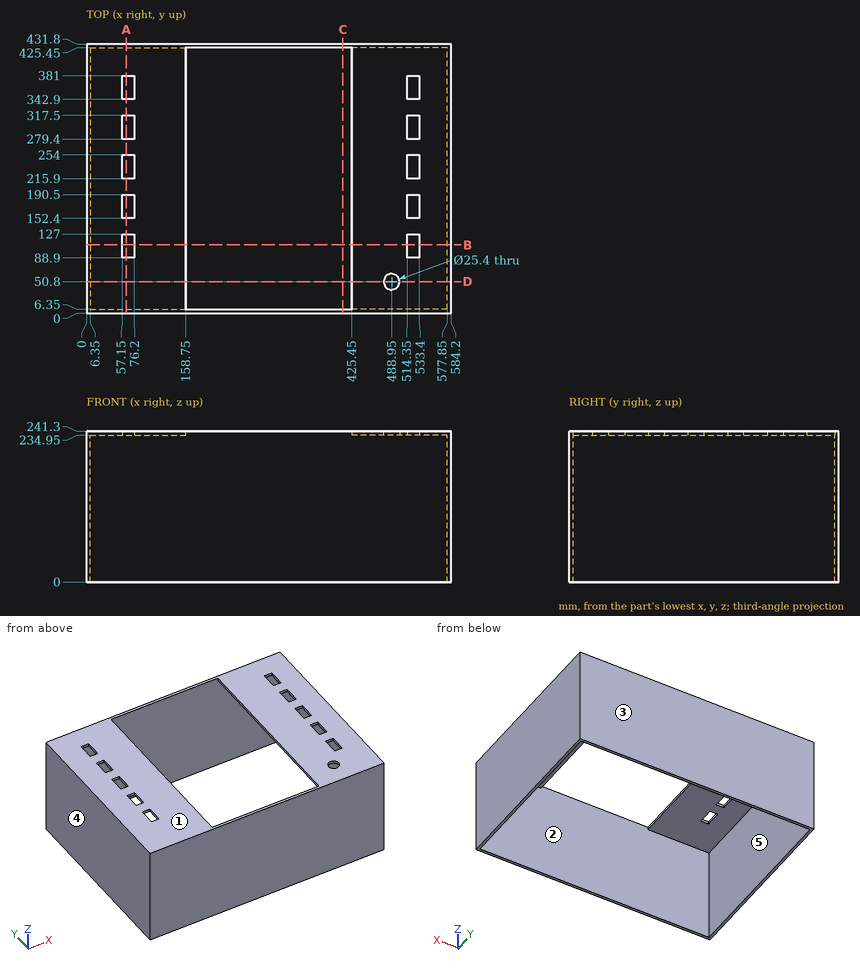
Geometry check sheet. Reference: drawing and pictorial views, mm from the part's lowest x, y, z. A direction names the side the tool comes from. Give positions to 0.01 mm unless a question says otherwise; leave off trailing zeros. Order: outer loops, then holes, each group sorted by start corner. A loop starts at its lowest first (then second) coordinate and runs counter-clockwise, first axis right, second up. Notation, with made-up numbers: M 2.5,61 L 32.5,61 A22 ccw 32.5,92 Z; hole C -3.5,11.5 d6. An arc over 180 degrees is marked long. Answer as a JSON object with one key per item and string values. Group by question number.
1) Cross-section at B-B (y = 110). Enter the section's corners in (x, z), then the cut area to 3 significant figures.
2) Depth check by flat-ended pin: pin 1 Ø3 at (y, z) = (120, 85) entering from -X; pin 2 Ø12 at (x, y) = (454.5, 231.5) entering from -Z. Enter the tip coordinate at first touch or a pass-through.
3) Cross-section at C-C (x = 411). Enter the section's corners in (y, z).
4) Mould release check, pull along Y, two halves, no side actions. Record for the marked faces 1, 2 and 3: released by +Y, released by -Y, zero draft, split by the parting line, or undercut.
5) Scan lines: line 1 along X through (y, z) = (50, 239); line 2 along X through (y, z) = (89, 194); line 3 along Y through (x, z) = (146.5, 23.5). Record each from-to range of solid material in increasing order. Write a range as [from, to].
6) Cross-section at A-A (x = 64). Enter the section's corners in (y, z).
7) Access from +Z, -Z, +X, -X, +Y, -Y to the whole of each face (thin tool, end or side, straight path). Record for the marked faces 4 and 5.
8) Cross-section at D-D (y = 50.8). Enter the section's corners in (x, z), then the cut area to 3 significant figures.
Result sheet:
{
 "1": {"outline": "M 0,0 L 6.35,0 L 6.35,234.95 L 57.15,234.95 L 57.15,241.3 L 0,241.3 Z; M 76.2,234.95 L 158.75,234.95 L 158.75,241.3 L 76.2,241.3 Z; M 425.45,234.95 L 514.35,234.95 L 514.35,241.3 L 425.45,241.3 Z; M 533.4,234.95 L 577.85,234.95 L 577.85,0 L 584.2,0 L 584.2,241.3 L 533.4,241.3 Z", "area": "4,760 mm2"},
 "2": {"pin 1": "stops at x = 0", "pin 2": "stops at z = 234.95"},
 "3": {"outline": "M 0,0 L 6.35,0 L 6.35,241.3 L 0,241.3 Z; M 425.45,0 L 431.8,0 L 431.8,241.3 L 425.45,241.3 Z"},
 "4": {"face 1": "zero draft", "face 2": "undercut", "face 3": "released by +Y"},
 "5": {"line 1": "x = [0, 158.75], [425.45, 476.28], [501.62, 584.2]", "line 2": "x = [0, 6.35], [577.85, 584.2]", "line 3": "y = [0, 6.35], [425.45, 431.8]"},
 "6": {"outline": "M 0,0 L 6.35,0 L 6.35,234.95 L 88.9,234.95 L 88.9,241.3 L 0,241.3 Z; M 127,234.95 L 152.4,234.95 L 152.4,241.3 L 127,241.3 Z; M 190.5,234.95 L 215.9,234.95 L 215.9,241.3 L 190.5,241.3 Z; M 254,234.95 L 279.4,234.95 L 279.4,241.3 L 254,241.3 Z; M 317.5,234.95 L 342.9,234.95 L 342.9,241.3 L 317.5,241.3 Z; M 381,234.95 L 425.45,234.95 L 425.45,0 L 431.8,0 L 431.8,241.3 L 381,241.3 Z"},
 "7": {"face 4": "+Z, -Z, -X, +Y, -Y", "face 5": "-Z"},
 "8": {"outline": "M 0,0 L 6.35,0 L 6.35,234.95 L 158.75,234.95 L 158.75,241.3 L 0,241.3 Z; M 425.45,234.95 L 476.25,234.95 L 476.25,241.3 L 425.45,241.3 Z; M 501.65,234.95 L 577.85,234.95 L 577.85,0 L 584.2,0 L 584.2,241.3 L 501.65,241.3 Z", "area": "4,840 mm2"}
}
